Autodesk Inventor part; units mm, degrees
ref_plane "Start Plane" through (0, 0, 19.2607) normal (0, 0, 1) x (1, 0, 0)
ref_plane "End Plane" through (0, 0, 1001.9635) normal (0, 0, 1) x (1, 0, 0)
ref_plane "Work Plane4" through (-2322.8437, 0, 140.6527) normal (-0.3457054, 0, 0.9383431) x (0.9383431, 0, 0.3457054)
ref_plane "Start Plane" through (0, 0, 19.2607) normal (0, 0, 1) x (1, 0, 0)
ref_plane "End Plane" through (0, 0, 1001.9635) normal (0, 0, 1) x (1, 0, 0)
sketch "Sketch" plane through (0, 0, 0) normal (0, 0, 1) x (1, 0, 0)
  line L0 (-15, -9) -> (-15, 9)
  line L1 (-9, 15) -> (9, 15)
  line L2 (15, 9) -> (15, -9)
  line L3 (9, -15) -> (-9, -15)
  arc A0 (-15, -9) -> (-9, -15) centre (-9, -9) ccw
  arc A1 (-9, 15) -> (-15, 9) centre (-9, 9) ccw
  arc A2 (15, 9) -> (9, 15) centre (9, 9) ccw
  arc A3 (9, -15) -> (15, -9) centre (9, -9) ccw
  arc A4 (-9, 12) -> (-12, 9) centre (-9, 9) ccw
  line L4 (-9, 12) -> (9, 12)
  arc A5 (12, 9) -> (9, 12) centre (9, 9) ccw
  line L5 (12, 9) -> (12, -9)
  arc A6 (9, -12) -> (12, -9) centre (9, -9) ccw
  line L6 (9, -12) -> (-9, -12)
  arc A7 (-12, -9) -> (-9, -12) centre (-9, -9) ccw
  line L7 (-12, -9) -> (-12, 9)
  line L8 (0, 22.7397) -> (0, -22.7397) construction
  line L9 (-22.7397, 0) -> (22.7397, 0) construction
  dimension "d7" = 6
  dimension "d10" = 30
  dimension "d11" = 30
  dimension "d12" = 3
  dimension "d15" = 15
  dimension "d16" = 15
extrude "Body" add sketch "Sketch" along normal up to surface (982.7028 mm away) from surface at 19.2607
sketch "Sketch3" plane through (0, 0, 0) normal (0, 0, 1) x (1, 0, 0)
  line L0 (0, 0) -> (10, 0)
ref_plane "Work Plane3" through (0, 0, 0) normal (0, -1, 0) x (1, 0, 0)
ref_plane "Work Plane4" through (-2322.8437, 0, 140.6527) normal (-0.3457054, 0, 0.9383431) x (0.9383431, 0, 0.3457054)
split "Split1" plane through (-2322.8437, 0, 140.6527) removes the side toward (-0.3457054, 0, 0.9383431)
ref_plane "Work Plane5" through (-380.5228, 991, -124.207) normal (0.3457054, 0, -0.9383431) x (-0.9383431, 0, -0.3457054)
split "Split2" plane through (-380.5228, 991, -124.207) removes the side toward (0.3457054, 0, -0.9383431)
ref_plane "Work Plane6" through (-314.3449, -9, 896.6115) normal (-0.9383431, 0, -0.3457054) x (-0.3457054, 0, 0.9383431)
split "Split3" plane through (-314.3449, -9, 896.6115) removes the side toward (-0.9383431, 0, -0.3457054)
sketch "Sketch4" plane through (0, 0, 0) normal (0, -1, 0) x (1, 0, 0)
  line L0 (-2, 19.2607) -> (12, 19.2607)
  line L1 (-2, 1001.9635) -> (12, 1001.9635)
  dimension "d18" = 982.7028
equation "\"d7\" = G_IR"
equation "\"d10\" = G_H"
equation "\"d11\" = G_W"
equation "\"d12\" = G_T"
equation "\"d15\" = 0.5 * d10"
equation "\"d16\" = 0.5 * d11"
equation "\"d3\" = G_L"
equation "\"G_W\" = 30"
equation "\"G_H\" = 30"
equation "\"G_T\" = 3"
equation "\"G_IR\" = 6"
equation "\"G_L\" = d18"
equation "\"G_OFFSET_START\" = -19.26073"
equation "\"G_OFFSET_END\" = -10.45931"
equation "\"d13\" = -G_OFFSET_START"
equation "\"d14\" = G_OFFSET_END + B_L"
equation "\"B_L\" = 1012.42284"
properties part number "DIN EN 10219-2 - 30 x 30 x 3  - 982.7" material "Steel, Mild"
Check sheet for the modelled part. Datum: model origin and axes. Units: mm. A direction names the side the tool comes from. Give positions to 0.01 mm unless a question says otherwise; leave off trailing zeros. Loops run counter-clockwise (first coordinate to the right, second up) from the corner with the lowest first, then second, coordinate; pieces in that order, holes last. Notation, with made-up numbers: M 58,24 L 100,24 A11 ccw 100,36 Z; hole C 58.5,2 d3. An arc over 180 degrees is marked long. Answer as CSV lines item,"result".
Item 1: Sectioned sample at A-A, the plane z = 582. Enter the section's corners in (x, y).
Reply:
outline,"M -15,-9 A6 ccw -9,-15 L 9,-15 A6 ccw 15,-9 L 15,9 A6 ccw 9,15 L -9,15 A6 ccw -15,9 Z; hole M -12,-9 A3 ccw -9,-12 L 9,-12 A3 ccw 12,-9 L 12,9 A3 ccw 9,12 L -9,12 A3 ccw -12,9 Z"
Item 2: Draft check along X on faces 3 (the face through (0, 15, 503)), 4 (the face through (-12, 0, 528)), 5 (the face through (-5.765, 12.152, 59.039)), 6 (the face through (0, 12, 503)). Enter one of: pulls with the +X half, pulls with the -X half, needs draft (parallel to the pull), parting line crosses it, or undercut.
Reply:
face 3,"needs draft"
face 4,"undercut"
face 5,"pulls with the -X half"
face 6,"undercut"
Item 3: Scan lines: L1, parallel to Y at x = -7.5, z = 122; L2, parallel to X at y = 10, z = 332. Record each from-to range of solid material in increasing order.
Reply:
L1,"-15 to -12, 12 to 15"
L2,"-14.92 to -11.83, 11.83 to 14.92"
Item 4: Depth check by flat-ended pin: pin 1 Ø3 at (x, y) = (2.5, 11) entering from +Z; pin 2 Ø6 at (x, y) = (-9.5, 5.5) entering from +Z; pin 3 Ø5 at (x, y) = (-4, -9) entering from +Z; pin 4 Ø2 at (x, y) = (4, 11.5) entering from +Z. Enter the tip coordinate at first touch or a pass-through.
Reply:
pin 1,"z = 997.77"
pin 2,"z = 992.02"
pin 3,"through"
pin 4,"z = 998.23"
Item 5: Sectioned sample at B-B, the plane x = -1.5. Enter the section's corners in (y, z), then the cut area to 3 significant figures.
Reply:
outline,"M -15,47.46 L -12,47.46 L -12,995.88 L -15,995.88 Z; M 12,47.46 L 15,47.46 L 15,995.88 L 12,995.88 Z"
area,"5,690 mm^2"
Item 6: Set-up check for faces 1 (the face through (12, 0, 504)), 2 (the face through (15, 0, 505)): record each of +Z, -Z, +X, -X, +Y, -Y from which the full face is reachable in a straight line by a thin tool's end or side.
Reply:
face 1,"+Z, -Z"
face 2,"+Z, -Z, +X, +Y, -Y"
